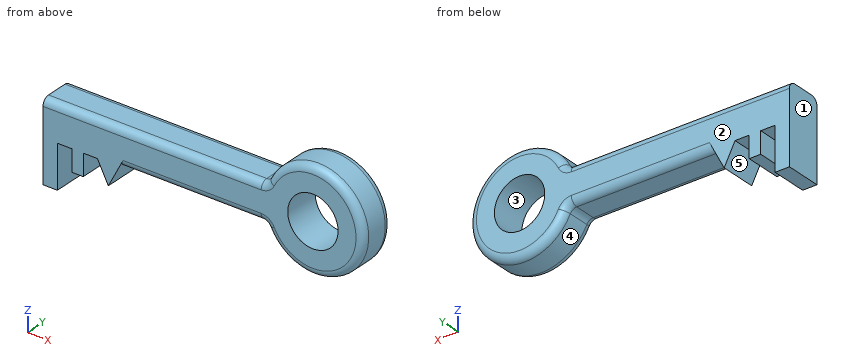
```python
from build123d import *

# Parameters (mm, degrees)
F0_R     = 17.5
F0_W     = 10
F0_H     = 30
F0_W_2   = 8
F0_H_2   = 15
F1_DEPTH = 25
F2_F1_R  = 5
F2_F2_R  = 5


with BuildPart() as f1:
    # F0 (on Front) → F1 (new body)
    with BuildSketch(Plane.XZ):
        with BuildLine():
            Line((-76.905815019, -12.5), (25.0358718634, -12.5))
            ThreePointArc((25.0358718634, -12.5), (92.7276139399, 0), (25.0358718634, 12.5))
            Line((25.0358718634, 12.5), (-129.9641281366, 12.5))
            Line((-129.9641281366, 12.5), (-129.9641281366, -12.5))
            Line((-129.9641281366, -12.5), (-119.9641281366, -12.5))
            Line((-119.9641281366, -12.5), (-109.9641281366, -12.5))
            Line((-109.9641281366, -12.5), (-101.9641281366, -12.5))
            Line((-101.9641281366, -12.5), (-92.1254744445, -12.5))
            Line((-92.1254744445, -12.5), (-76.905815019, -12.5))
        make_face()
        with Locations((57.7276139399, 0)):
            Circle(F0_R, mode=Mode.SUBTRACT)
        with Locations((-124.9641281366, -27.5)):
            Rectangle(F0_W, F0_H)
        with Locations((-105.9641281366, -20)):
            Rectangle(F0_W_2, F0_H_2)
        Polygon((-84.5156447317, -27.2000782564), (-76.905815019, -12.5), (-92.1254744445, -12.5), align=None)
    extrude(amount=F1_DEPTH)

    # F2: fillet of radius 5 on 4 edges, made by hand

    # F2_f1
    f2_f1_edges = [f1.edges().sort_by_distance(p)[0] for p in [
        (25.0358718634, -12.5, -12.5),
        (25.0358718634, -12.5, 12.5),
    ]]
    fillet(f2_f1_edges, radius=F2_F1_R)

    # F2_f2
    f2_f2_edges = [f1.edges().sort_by_distance(p)[0] for p in [
        (92.7276139399, 0, 0),
        (92.7276139399, -25, 0),
        (24.4105279445, -25, -13.2610437605),
        (24.4105279445, -25, 13.2610437605),
        (24.4105279445, 0, -13.2610437605),
        (24.4105279445, 0, 13.2610437605),
    ]]
    fillet(f2_f2_edges, radius=F2_F2_R)


solid = f1.part
```
For this review, take the finished solid that the model builds, in its own axes (mm). Face numbers are marked on the shaded views. A direction names the side the tool comes from. Round coordinates to 2 decimals unless told otherwise and drop trailing zeros. Write each loop counter-clockwise with the first axis right and the second up, starting at its lowest first coordinate (ties: lowest second). Pieces come first, ordered by that corner, then holes. Notation, with made-up numbers: (-8.5, 81) - (43.5, 81) arc R7 cw to (43.5, 92) - close; hole circle Ø11 at (34, -37). An arc over 180 degrees is marked (long way). Put each result on its own line as item: value.
Q1. We need section C-C (x = -82). Give the boundary of the cut face in (y, z), and give its area (3 significant figures).
Solved:
outline: (-25, -22.34) - (0, -22.34) - (0, 7.5) arc R5 ccw to (-5, 12.5) - (-20, 12.5) arc R5 ccw to (-25, 7.5) - close
area: 860 mm2
Q2. Insertion check: pin 1 Ø4 at (x, y) = (-105, -15.5) entering from -Z; pin 2 Ø4.5 at (x, y) = (-40, -11) entering from -Z; pin 3 Ø4 at (x, y) = (39, -12.5) entering from -Z. Each pin has a flat end and moves straight along its axis. Give the tip position at first contact, or say it passes through.
Solved:
pin 1: stops at z = -27.5
pin 2: stops at z = -12.5
pin 3: stops at z = -30.74
Q3. Mouldability with a two-part tool opening along X and no side actions: class the marked faces 1, 2 and 3 as released by +X, released by -X, zero draft, split by the parting line, or undercut.
Solved:
face 1: released by -X
face 2: zero draft
face 3: undercut
Q4. Wall thickness on probe 1 along X at (y, z) = (-1.25, -15); probe 2 along X at (y, z) = (-4.5, -35.5); probe 3 along X at (y, z) = (-5, -11): over which ranges is each line inside the solid? List them lowest first.
Solved:
probe 1: x = -129.96 to -119.96, -109.96 to -101.96, -90.83 to -78.2, 27.99 to 48.71, 66.74 to 87.47
probe 2: x = -129.96 to -119.96
probe 3: x = -129.96 to 44.12, 71.34 to 90.95
Q5. We need section B-B (x = -16.5). Give the boundary of the cut face in (y, z), and give its area (3 significant figures).
Solved:
outline: (-25, -7.5) arc R5 ccw to (-20, -12.5) - (-5, -12.5) arc R5 ccw to (0, -7.5) - (0, 7.5) arc R5 ccw to (-5, 12.5) - (-20, 12.5) arc R5 ccw to (-25, 7.5) - close
area: 604 mm2
Q6. We need section A-A (y = -17). Give the boundary of the cut face in (x, z).
Solved:
outline: (-129.96, -42.5) - (-119.96, -42.5) - (-119.96, -12.5) - (-109.96, -12.5) - (-109.96, -27.5) - (-101.96, -27.5) - (-101.96, -12.5) - (-92.13, -12.5) - (-84.52, -27.2) - (-76.91, -12.5) - (21.76, -12.5) arc R5 cw to (26.25, -15.31) arc R35 ccw (long way) to (26.25, 15.31) arc R5 cw to (21.76, 12.5) - (-129.96, 12.5) - close; hole circle Ø35 at (57.73, 0)
Q7. Machinability: for the marked faces 4 and 5, which of the approach directions +Z, -Z, +X, -X, +Y, -Y give a long, thin tool a straight path to every point of the face, cutting with its end or side? Answer none if there is none.
Solved:
face 4: +Y, -Y
face 5: -Z, +Y, -Y
